from build123d import *

# Parameters (mm, degrees)
SKETCH1_W                 = 215.08
SKETCH1_H                 = 78.74
BOSS_EXTRUDE1_DEPTH       = 0.508
SKETCH1_3_W               = 215.08
SKETCH1_3_H               = 8.255
SKETCH1_3_H_2             = 78.74
SKETCH1_3_W_2             = 210
SKETCH1_3_H_3             = 73.66
BOSS_EXTRUDE2_DEPTH       = 27
BOSS_EXTRUDE3_START       = 21.59
BOSS_EXTRUDE3_DEPTH       = 32.5
SKETCH1_4_W               = 215.08
SKETCH1_4_H               = 8.255
BOSS_EXTRUDE4_DEPTH       = 0.508
F_4_40_TAPPED_HOLE2_D     = 2.2606
F_4_40_TAPPED_HOLE2_DEPTH = 7.62
F_4_40_TAPPED_HOLE2_TIP   = 0.679152758
SKETCH13_W                = 141.42
SKETCH13_H                = 8.255
SKETCH13_W_2              = 26.67
CUT_EXTRUDE1_DEPTH        = 28.508


with BuildPart() as part:
    # Sketch1 → Boss-Extrude1 (new body)
    with BuildSketch(Plane(origin=(0, 0, 0), x_dir=(1, 0, 0), z_dir=(0, 1, 0))):
        with Locations((107.54, -39.37)):
            Rectangle(SKETCH1_W, SKETCH1_H)
    extrude(amount=-BOSS_EXTRUDE1_DEPTH)

    # Sketch1<3> → Boss-Extrude2 (add)
    with BuildSketch(Plane(origin=(0, 0, 0), x_dir=(1, 0, 0), z_dir=(0, 1, 0))):
        with Locations((107.54, 4.1275)):
            Rectangle(SKETCH1_3_W, SKETCH1_3_H)
        with Locations((107.54, -82.8675)):
            Rectangle(SKETCH1_3_W, SKETCH1_3_H)
        with Locations((107.54, -39.37)):
            Rectangle(SKETCH1_3_W, SKETCH1_3_H_2)
        with Locations((107.54, -39.37)):
            Rectangle(SKETCH1_3_W_2, SKETCH1_3_H_3, mode=Mode.SUBTRACT)
    extrude(amount=BOSS_EXTRUDE2_DEPTH)

    # Sketch5 → Boss-Extrude3 (add)
    with BuildSketch(Plane.XY.offset(2.54).offset(BOSS_EXTRUDE3_START)):
        with BuildLine():
            Line((29.54, 7), (27.54, 7))
            ThreePointArc((27.54, 7), (23.600043647, 1.985651932), (17.54, 0))
            Line((17.54, 0), (39.54, 0))
            ThreePointArc((39.54, 0), (33.479956353, 1.985651932), (29.54, 7))
        make_face()
        with BuildLine():
            Line((55.4988, 7), (53.4988, 7))
            ThreePointArc((53.4988, 7), (49.558843647, 1.985651932), (43.4988, 0))
            Line((43.4988, 0), (65.4988, 0))
            ThreePointArc((65.4988, 0), (59.438756353, 1.985651932), (55.4988, 7))
        make_face()
        with BuildLine():
            Line((81.4576, 7), (79.4576, 7))
            ThreePointArc((79.4576, 7), (75.517643647, 1.985651932), (69.4576, 0))
            Line((69.4576, 0), (91.4576, 0))
            ThreePointArc((91.4576, 0), (85.397556353, 1.985651932), (81.4576, 7))
        make_face()
        with BuildLine():
            Line((107.4164, 7), (105.4164, 7))
            ThreePointArc((105.4164, 7), (101.476443647, 1.985651932), (95.4164, 0))
            Line((95.4164, 0), (117.4164, 0))
            ThreePointArc((117.4164, 0), (111.356356353, 1.985651932), (107.4164, 7))
        make_face()
        with BuildLine():
            Line((133.3752, 7), (131.3752, 7))
            ThreePointArc((131.3752, 7), (127.435243647, 1.985651932), (121.3752, 0))
            Line((121.3752, 0), (143.3752, 0))
            ThreePointArc((143.3752, 0), (137.315156353, 1.985651932), (133.3752, 7))
        make_face()
        with BuildLine():
            Line((159.334, 7), (157.334, 7))
            ThreePointArc((157.334, 7), (153.394043647, 1.985651932), (147.334, 0))
            Line((147.334, 0), (169.334, 0))
            ThreePointArc((169.334, 0), (163.273956353, 1.985651932), (159.334, 7))
        make_face()
        with BuildLine():
            Line((185.2928, 7), (183.2928, 7))
            ThreePointArc((183.2928, 7), (179.352843647, 1.985651932), (173.2928, 0))
            Line((173.2928, 0), (195.2928, 0))
            ThreePointArc((195.2928, 0), (189.232756353, 1.985651932), (185.2928, 7))
        make_face()
    extrude(amount=BOSS_EXTRUDE3_DEPTH)

    # Sketch1<4> → Boss-Extrude4 (add)
    with BuildSketch(Plane(origin=(0, 0, 0), x_dir=(1, 0, 0), z_dir=(0, 1, 0))):
        with Locations((107.54, 4.1275)):
            Rectangle(SKETCH1_4_W, SKETCH1_4_H)
        with Locations((107.54, -82.8675)):
            Rectangle(SKETCH1_4_W, SKETCH1_4_H)
    extrude(amount=-BOSS_EXTRUDE4_DEPTH)

    # #4-40 Tapped Hole2
    with Locations(Plane(origin=(0, 27, 0), x_dir=(-1, 0, 0), z_dir=(0, 1, 0))):
        with Locations((-31.75, 0), (-183.33, 0), (-31.75, 78.74), (-183.33, 78.74)):
            Hole(F_4_40_TAPPED_HOLE2_D / 2, depth=F_4_40_TAPPED_HOLE2_DEPTH)
            with Locations((0, 0, -(F_4_40_TAPPED_HOLE2_DEPTH + F_4_40_TAPPED_HOLE2_TIP / 2))):  # 118° drill point
                Cone(0, F_4_40_TAPPED_HOLE2_D / 2, F_4_40_TAPPED_HOLE2_TIP, mode=Mode.SUBTRACT)

    # Sketch13 → Cut-Extrude1 (cut, through all)
    with BuildSketch(Plane(origin=(0, 27, 0), x_dir=(1, 0, 0), z_dir=(0, 1, 0))):
        with Locations((107.54, 4.1275)):
            Rectangle(SKETCH13_W, SKETCH13_H)
        with Locations((107.54, -82.8675)):
            Rectangle(SKETCH13_W, SKETCH13_H)
        with Locations((13.335, 4.1275)):
            Rectangle(SKETCH13_W_2, SKETCH13_H)
        with Locations((201.745, 4.1275)):
            Rectangle(SKETCH13_W_2, SKETCH13_H)
        with Locations((201.745, -82.8675)):
            Rectangle(SKETCH13_W_2, SKETCH13_H)
        with Locations((13.335, -82.8675)):
            Rectangle(SKETCH13_W_2, SKETCH13_H)
    extrude(amount=-CUT_EXTRUDE1_DEPTH, mode=Mode.SUBTRACT)


solid = part.part
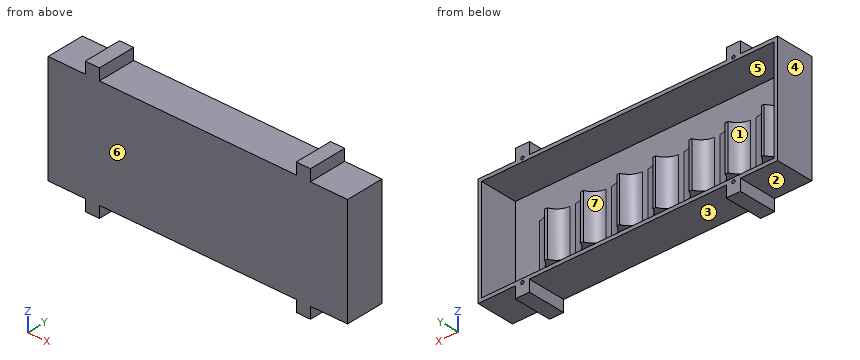
Model file for the job. Use its own axes, mm. Face numbers are marked on the shaded views. A direction names the side the tool comes from. Give positions to 0.01 mm unless a question says otherwise; leave off trailing zeros. Order: outer loops, then holes, each group sorted by start corner. A loop starts at its lowest first (then second) coordinate and runs counter-clockwise, first axis right, second up. Notation, with made-up numbers: (24, 85) - (79, 85) arc R26 ccw to (79, 120) - close; hole circle Ø10 at (-5, 1). An arc over 180 degrees is marked (long way). One line per item, written item: value.
Item 1: Wall check: line 1 (Z direction, x = 31.75, y = 23.25) (3 decimals); line 2 (Z direction, x = 147.5, y = 5.75); line 3 (X direction, y = 5, z = 67). Give the ranges that are in metal, low to high.
Response values:
line 1: -8.255 to -1.13, 1.13 to 2.54, 76.2 to 77.61, 79.87 to 86.995
line 2: 0 to 2.54, 76.2 to 78.74
line 3: 0 to 2.54, 212.54 to 215.08
Item 2: Slice it at D-D (x = 75). List the corners of the cut face in (y, z), then the cut area to 3 significant figures.
Response values:
outline: (-0.51, 0) - (27, 0) - (27, 2.54) - (0, 2.54) - (0, 24.13) - (1.64, 24.13) - (1.64, 56.63) - (0, 56.63) - (0, 76.2) - (27, 76.2) - (27, 78.74) - (-0.51, 78.74) - close
area: 231 mm2
Item 3: Slice it at B-B (z = 6). List the corners of the cut face in (x, y), then the cut area to 3 significant figures.
Response values:
outline: (0, -0.51) - (215.08, -0.51) - (215.08, 27) - (212.54, 27) - (212.54, 0) - (2.54, 0) - (2.54, 27) - (0, 27) - close
area: 246 mm2
Item 4: Two-plate mould, pull along X, no slides. Class the marked faces 4, 5, 6 and 7: released by +X, released by -X, zero draft, split by the parting line, or undercut.
Response values:
face 4: released by -X
face 5: undercut
face 6: zero draft
face 7: undercut
Item 5: Tool access for the marked faces 1, 2 and 3: list every direction of +Z, -Z, +X, -X, +Y, -Y with a clear straight run to the whole face (end or side of a thin tool).
Response values:
face 1: +Y
face 2: -Z, -X, +Y, -Y
face 3: -Z, +Y, -Y
Item 6: Pin check, flat tips, straight feed: pin 1 Ø7.5 at (x, y) = (106.5, 2.5) entering from -Z; pin 2 Ø2.5 at (y, z) = (9.5, 83.5) entering from +X; pin 3 Ø7.5 at (x, y) = (109.5, 4.5) entering from +Z. Stop position of each tip, or through.
Response values:
pin 1: z = 0
pin 2: x = 188.41
pin 3: z = 78.74
Item 7: Slice it at A-A (y = 24.5). List the corners of the cut face in (x, z) (3 decimals), then the cut area to 3 significant figures.
Response values:
outline: (0, 0) - (26.67, 0) - (26.67, -8.255) - (36.83, -8.255) - (36.83, 0) - (178.25, 0) - (178.25, -8.255) - (188.41, -8.255) - (188.41, 0) - (215.08, 0) - (215.08, 78.74) - (188.41, 78.74) - (188.41, 86.995) - (178.25, 86.995) - (178.25, 78.74) - (36.83, 78.74) - (36.83, 86.995) - (26.67, 86.995) - (26.67, 78.74) - (0, 78.74) - close; hole (2.54, 2.54) - (212.54, 2.54) - (212.54, 76.2) - (2.54, 76.2) - close; hole circle Ø2.261 at (31.75, 0); hole circle Ø2.261 at (31.75, 78.74); hole circle Ø2.261 at (183.33, 0); hole circle Ø2.261 at (183.33, 78.74)
area: 1,790 mm2
Item 8: Slice it at C-C (y = 9.5). List the corners of the cut face in (x, z) (3 decimals), then the cut area to 3 significant figures.
Response values:
outline: (0, 0) - (26.67, 0) - (26.67, -8.255) - (36.83, -8.255) - (36.83, 0) - (178.25, 0) - (178.25, -8.255) - (188.41, -8.255) - (188.41, 0) - (215.08, 0) - (215.08, 78.74) - (188.41, 78.74) - (188.41, 86.995) - (178.25, 86.995) - (178.25, 78.74) - (36.83, 78.74) - (36.83, 86.995) - (26.67, 86.995) - (26.67, 78.74) - (0, 78.74) - close; hole (2.54, 2.54) - (212.54, 2.54) - (212.54, 76.2) - (2.54, 76.2) - close
area: 1,800 mm2
